The listing builds one solid part. Answer for the finished solid, in the listing's coordinates (mm). Coordinates: 2 decimals unless noted, no trailing zeros. Loops run counter-clockwise (first coordinate to the right, second up) from the corner with the lowest first, then second, coordinate; pieces in that order, holes last. Notation, with made-up numbers: (-7.75, 15.5) -> (-2.75, 15.5) arc R26 ccw to (-2.75, 31.5) -> close; hole circle Ø10 at (-19.5, 46.25). An arc over 180 degrees is marked (long way). Answer in a Markdown table with one row per item.
```python
from build123d import *

# Parameters (mm, degrees)
F1_DEPTH = 1219.2
F2_R     = 0.79375
F3_R     = 1.5875


# Not quite as in the source:
# - a feature names something its author has since deleted; it is built from what else it names


with BuildPart() as f1:
    # F0 (on Front) → F1 (new body)
    with BuildSketch(Plane.XZ):
        Polygon((-25.4, 0), (0, 0), (25.4, 0), (25.4, 12.7), (6.35, 12.7), (6.35, 11.1125), (23.8125, 11.1125), (23.8125, 1.5875), (0, 1.5875), (-23.8125, 1.5875), (-23.8125, 11.1125), (-6.35, 11.1125), (-6.35, 12.7), (-25.4, 12.7), align=None)
    extrude(amount=F1_DEPTH)

    # F2
    f2_edges = [f1.edges().sort_by_distance(p)[0] for p in [
        (-23.8125, -609.6, 1.5875),
        (-23.8125, -609.6, 11.1125),
        (23.8125, -609.6, 1.5875),
        (23.8125, -609.6, 11.1125),
    ]]
    fillet(f2_edges, radius=F2_R)

    # F3
    f3_edges = [f1.edges().sort_by_distance(p)[0] for p in [
        (25.4, -609.6, 12.7),
        (25.4, -609.6, 0),
        (-25.4, -609.6, 0),
        (-25.4, -609.6, 12.7),
    ]]
    fillet(f3_edges, radius=F3_R)


solid = f1.part
```
Item 1: Determine the mould class of faces 1 (the face through (0, -601, 0)), 2 (the face through (0, -601, 1.588)) for opening direction X: +X half, -X half, draft (parallel to the pull), parting line (faces both ways), or undercut.
Findings below:
| item | result |
|---|---|
| face 1 | draft |
| face 2 | undercut |
Item 2: A cutting plane is placed at A-A, the plane z = 5.25. Determine the outline of the cut face in (x, y).
Findings below:
| item | result |
|---|---|
| outline | (-25.4, -1219.2) -> (-23.81, -1219.2) -> (-23.81, 0) -> (-25.4, 0) -> close; (23.81, -1219.2) -> (25.4, -1219.2) -> (25.4, 0) -> (23.81, 0) -> close |
Item 3: Flat-ended cylindrical pins translate along their axes: pin 1 Ø1 at (x, z) = (-17.5, 10) entering from +Y; pin 2 Ø0.5 at (y, z) = (-380, 12) entering from +X. Find the tip coordinate at first contact, or state that the pin passes through.
Findings below:
| item | result |
|---|---|
| pin 1 | passes through |
| pin 2 | stops at x = 25.27 |
Item 4: Find the intervals of material crossed by probe 1 along X at (y, z) = (-1111, 8); probe 2 along Z at (x, y) = (-12.5, -900); probe 3 along X at (y, z) = (-426, 2), in increasing order.
Findings below:
| item | result |
|---|---|
| probe 1 | x = -25.4 to -23.81, 23.81 to 25.4 |
| probe 2 | z = 0 to 1.59, 11.11 to 12.7 |
| probe 3 | x = -25.4 to -23.71, 23.71 to 25.4 |
